Read the model definition and answer for the solid it produces. Units are mm, in the model's axes. Face numbers are marked on the shaded views. A direction names the side the tool comes from. Give positions to 0.01 mm unless a question says otherwise; leave off trailing zeros. Order: outer loops, then holes, each group sorted by start corner. A loop starts at its lowest first (then second) coordinate and runs counter-clockwise, first axis right, second up.
```python
from build123d import *

# Parameters (mm, degrees)
SCHIZZO2_W                                           = 51.888116
SCHIZZO2_H                                           = 40
ESTRUSIONE_ESTRUSIONE2_DEPTH                         = 10
ESTRUSIONE_ESTRUSIONE3_DEPTH                         = 12.5
ESTRUSIONE_ESTRUSIONE3_DEPTH_BACK                    = 10
SCHIZZO3_R                                           = 113
SCHIZZO3_R_2                                         = 105
SCHIZZO3_R_3                                         = 95
SCHIZZO3_R_4                                         = 92.5
TAGLIO_ESTRUSIONE1_DEPTH                             = 4.5
TAGLIO_ESTRUSIONE1_DEPTH_BACK                        = 4.5
SCHIZZO3_3_R                                         = 115
SCHIZZO3_3_R_2                                       = 113
SCHIZZO3_3_R_3                                       = 105
SCHIZZO3_3_R_4                                       = 95
TAGLIO_ESTRUSIONE2_DEPTH                             = 12.5
TAGLIO_ESTRUSIONE2_DEPTH_BACK                        = 12.5
SCHIZZO3_4_R                                         = 121.5
SCHIZZO3_4_R_2                                       = 115
TAGLIO_ESTRUSIONE3_DEPTH                             = 79.5
TAGLIO_ESTRUSIONE3_DEPTH_BACK                        = 79.5
ESTRUSIONE_ESTRUSIONE5_DEPTH                         = 51.888111
FORO_LAMATO_PER_VITE_M4_A_TESTA_CILINDRI_D           = 4.5
FORO_LAMATO_PER_VITE_M4_A_TESTA_CILINDRI_DEPTH       = 30
FORO_LAMATO_PER_VITE_M4_A_TESTA_CILINDRI_CBORE_D     = 10
FORO_LAMATO_PER_VITE_M4_A_TESTA_CILINDRI_CBORE_DEPTH = 2.6
FORO_LAMATO_PER_VITE_M4_A_TESTA_CILINDRI_TIP         = 1.351936393
SCHIZZO10_W                                          = 2
SCHIZZO10_H                                          = 17
TAGLIO_ESTRUSIONE4_DEPTH                             = 10
TAGLIO_ESTRUSIONE5_DEPTH                             = 33
RACCORDO1_R                                          = 10


with BuildPart() as part:
    # Schizzo2 → Estrusione-Estrusione2 (new body)
    with BuildSketch(Plane(origin=(0, 0, 0), x_dir=(1, 0, 0), z_dir=(0, 1, 0))):
        with Locations((-97.308977, 0)):
            Rectangle(SCHIZZO2_W, SCHIZZO2_H)
    extrude(amount=-ESTRUSIONE_ESTRUSIONE2_DEPTH)

    # Schizzo3 → Estrusione-Estrusione3 (add, two sides: drawn at the far end of the back side and taken through both)
    # profile 1 of 3: a face of its own
    with BuildSketch(Plane.XY.offset(-ESTRUSIONE_ESTRUSIONE3_DEPTH_BACK)):
        with Locations((0, 44)):
            Circle(SCHIZZO3_R)
        with Locations((0, 44)):
            Circle(SCHIZZO3_R_2, mode=Mode.SUBTRACT)
    # profile 2 of 3: a face of its own
    with BuildSketch(Plane.XY.offset(-ESTRUSIONE_ESTRUSIONE3_DEPTH_BACK)):
        with Locations((0, 44)):
            Circle(SCHIZZO3_R_2)
        with Locations((0, 44)):
            Circle(SCHIZZO3_R_3, mode=Mode.SUBTRACT)
    # profile 3 of 3: a face of its own
    with BuildSketch(Plane.XY.offset(-ESTRUSIONE_ESTRUSIONE3_DEPTH_BACK)):
        with Locations((0, 44)):
            Circle(SCHIZZO3_R_3)
        with Locations((0, 44)):
            Circle(SCHIZZO3_R_4, mode=Mode.SUBTRACT)
    extrude(amount=ESTRUSIONE_ESTRUSIONE3_DEPTH + ESTRUSIONE_ESTRUSIONE3_DEPTH_BACK)

    # Schizzo3<3> → Taglio-Estrusione1 (cut, two sides: drawn at the far end of the back side and taken through both)
    # profile 1 of 3: a face of its own
    with BuildSketch(Plane.XY.offset(-TAGLIO_ESTRUSIONE1_DEPTH_BACK)):
        with Locations((0, 44)):
            Circle(SCHIZZO3_3_R)
        with Locations((0, 44)):
            Circle(SCHIZZO3_3_R_2, mode=Mode.SUBTRACT)
    # profile 2 of 3: a face of its own
    with BuildSketch(Plane.XY.offset(-TAGLIO_ESTRUSIONE1_DEPTH_BACK)):
        with Locations((0, 44)):
            Circle(SCHIZZO3_3_R_2)
        with Locations((0, 44)):
            Circle(SCHIZZO3_3_R_3, mode=Mode.SUBTRACT)
    # profile 3 of 3: a face of its own
    with BuildSketch(Plane.XY.offset(-TAGLIO_ESTRUSIONE1_DEPTH_BACK)):
        with Locations((0, 44)):
            Circle(SCHIZZO3_3_R_3)
        with Locations((0, 44)):
            Circle(SCHIZZO3_3_R_4, mode=Mode.SUBTRACT)
    extrude(amount=TAGLIO_ESTRUSIONE1_DEPTH + TAGLIO_ESTRUSIONE1_DEPTH_BACK, mode=Mode.SUBTRACT)

    # Schizzo3<4> → Taglio-Estrusione2 (cut, two sides: drawn at the far end of the back side and taken through both)
    with BuildSketch(Plane.XY.offset(-TAGLIO_ESTRUSIONE2_DEPTH_BACK)):
        with Locations((0, 44)):
            Circle(SCHIZZO3_4_R)
        with Locations((0, 44)):
            Circle(SCHIZZO3_4_R_2, mode=Mode.SUBTRACT)
    extrude(amount=TAGLIO_ESTRUSIONE2_DEPTH + TAGLIO_ESTRUSIONE2_DEPTH_BACK, mode=Mode.SUBTRACT)

    # Schizzo4 → Taglio-Estrusione3 (cut, two sides: drawn at the far end of the back side and taken through both)
    with BuildSketch(Plane.XY.offset(12.5).offset(-TAGLIO_ESTRUSIONE3_DEPTH_BACK)):
        Polygon((150, 13), (150, -10), (150, -80), (-150, -80), (-150, -10), (0, -10), (0, 13), (-150, 13), (-150, 163), (150, 163), align=None)
    extrude(amount=TAGLIO_ESTRUSIONE3_DEPTH + TAGLIO_ESTRUSIONE3_DEPTH_BACK, mode=Mode.SUBTRACT)

    # Smusso1
    # the kernel refuses this chamfer: 4.942054941, 3 mm, written as the material it takes off along each edge
    with BuildSketch(Plane(origin=(-87.150731494, 13, 24.790313744), x_dir=(-0.998955732576957, 0.045688558213574655, 0), z_dir=(0, 0, -1))) as smusso1_piece_1:
        with BuildLine():
            Line((3.009603279, 0), (-2.049272113, -4.468643386))
            Line((-2.049272113, -4.468643386), (-2.138755111, -4.426662964))
            ThreePointArc((-2.138755111, -4.426662964), (-1.049342002, -2.223465239), (-0.091514438, 0.037345286))
            Line((-0.091514438, 0.037345286), (0.004515907, 0.098737882))
            ThreePointArc((0.004515907, 0.098737882), (1.506176357, 0.030057461), (3.014119187, 0.098737882))
            Line((3.014119187, 0.098737882), (3.009603279, 0))
        make_face()
    extrude(amount=47.080627488, mode=Mode.SUBTRACT)
    # the kernel refuses this chamfer: 4.942054941, 3 mm, written as the material it takes off along each edge
    with BuildSketch(Plane(origin=(-116.379670622, 13, -10), x_dir=(0, -0.9996219169112969, -0.02749587661058621), z_dir=(1, 0, 0))) as smusso1_2_piece_1:
        with BuildLine():
            Line((3.086019586, 0), (-0.169641465, -3.081353381))
            Line((-0.169641465, -3.081353381), (-0.22961878, -3.079703628))
            ThreePointArc((-0.22961878, -3.079703628), (-0.102387681, -1.540193489), (-0.059977315, 0.001649753))
            Line((-0.059977315, 0.001649753), (0.001649753, 0.059977315))
            ThreePointArc((0.001649753, 0.059977315), (1.543492994, 0.017566949), (3.087669338, 0.059977315))
            Line((3.087669338, 0.059977315), (3.086019586, 0))
        make_face()
    extrude(amount=34.07955152, mode=Mode.SUBTRACT)
    with BuildSketch(Plane(origin=(-116.379670622, 13, 12.5), x_dir=(0, -0.9996219169112969, 0.02749587661058621), z_dir=(1, 0, 0))) as smusso1_2_piece_2:
        with BuildLine():
            Line((3.086019586, 0), (-0.169641465, 3.081353381))
            Line((-0.169641465, 3.081353381), (-0.22961878, 3.079703628))
            ThreePointArc((-0.22961878, 3.079703628), (-0.102387681, 1.540193489), (-0.059977315, -0.001649753))
            Line((-0.059977315, -0.001649753), (0.001649753, -0.059977315))
            ThreePointArc((0.001649753, -0.059977315), (1.543492994, -0.017566949), (3.087669338, -0.059977315))
            Line((3.087669338, -0.059977315), (3.086019586, 0))
        make_face()
    extrude(amount=34.07955152, mode=Mode.SUBTRACT)

    # Schizzo7 → Estrusione-Estrusione5 (add)
    with BuildSketch(Plane(origin=(-71.364919, 0, 0), x_dir=(0, 0, -1), z_dir=(1, 0, 0))):
        Polygon((-20, 0), (-35, 0), (-35, 4), (-20, 4), (-14, 0), align=None)
        Polygon((20, 4), (35, 4), (35, 0), (20, 0), (14, 0), align=None)
    extrude(amount=-ESTRUSIONE_ESTRUSIONE5_DEPTH)

    # Foro lamato per Vite M4 a testa cilindrica piana-1
    with Locations(Plane(origin=(0, 4, 0), x_dir=(1, 0, 0), z_dir=(0, 1, 0))):
        with Locations((-97.308977, -27.5), (-97.308977, 27.5)):
            CounterBoreHole(FORO_LAMATO_PER_VITE_M4_A_TESTA_CILINDRI_D / 2, FORO_LAMATO_PER_VITE_M4_A_TESTA_CILINDRI_CBORE_D / 2, FORO_LAMATO_PER_VITE_M4_A_TESTA_CILINDRI_CBORE_DEPTH, depth=FORO_LAMATO_PER_VITE_M4_A_TESTA_CILINDRI_DEPTH)
            with Locations((0, 0, -(FORO_LAMATO_PER_VITE_M4_A_TESTA_CILINDRI_DEPTH + FORO_LAMATO_PER_VITE_M4_A_TESTA_CILINDRI_TIP / 2))):  # 118° drill point
                Cone(0, FORO_LAMATO_PER_VITE_M4_A_TESTA_CILINDRI_D / 2, FORO_LAMATO_PER_VITE_M4_A_TESTA_CILINDRI_TIP, mode=Mode.SUBTRACT)

    # Schizzo10 → Taglio-Estrusione4 (cut)
    with BuildSketch(Plane(origin=(0, 0, 0), x_dir=(1, 0, 0), z_dir=(0, 1, 0))):
        with Locations((-116.253035279, 0)):
            Rectangle(SCHIZZO10_W, SCHIZZO10_H)
    extrude(amount=-TAGLIO_ESTRUSIONE4_DEPTH, mode=Mode.SUBTRACT)

    # Schizzo11 → Taglio-Estrusione5 (cut)
    with BuildSketch(Plane(origin=(0, 4, 0), x_dir=(1, 0, 0), z_dir=(0, 1, 0))):
        Polygon((-123.253035, 14), (-123.253035, 35), (-104.808977, 35), (-114.808977, 14), align=None)
        Polygon((-89.808977, 35), (-71.364919, 35), (-71.364919, 14), (-79.808977, 14), align=None)
        Polygon((-123.253035, -14), (-123.253035, -35), (-104.808977, -35), (-114.808977, -14), align=None)
        Polygon((-89.808977, -35), (-71.364919, -35), (-71.364919, -14), (-79.808977, -14), align=None)
    extrude(amount=-TAGLIO_ESTRUSIONE5_DEPTH, mode=Mode.SUBTRACT)

    # Raccordo1
    raccordo1_edges = [part.edges().sort_by_distance(p)[0] for p in [
        (-104.808977, 2, -35),
        (-89.808977, 2, -35),
        (-104.808977, 2, 35),
        (-89.808977, 2, 35),
    ]]
    fillet(raccordo1_edges, radius=RACCORDO1_R)


solid = part.part
```
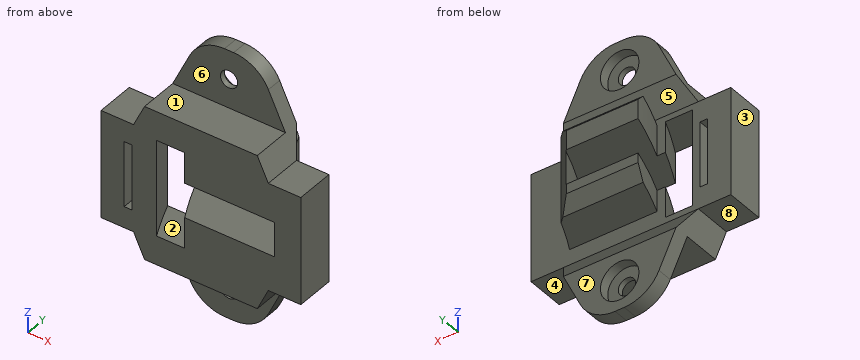
1) A tool of negligible diameter and unlimited length cuts with its end or side. For the marked faces 4, 5, 6, 7 and 8, from which of +Z, -Z, +X, -X, +Y, -Y can it reach the whole face along a straight path? Write none if from no direction.
Final values:
face 4: -Z, +X, +Y, -Y
face 5: +X, -X, +Y
face 6: +Z, +X, -X, -Y
face 7: -Z, +X, -X, +Y
face 8: -Z, -X, +Y, -Y
2) The part is cut by section C-C on z = -28.5. Determine the outline of the cut face in (x, y).
Final values:
outline: (-107.9, 0) - (-99.32, 0) - (-99.32, 1.4) - (-102.21, 1.4) - (-102.21, 4) - (-107.9, 4) - close; (-95.29, 0) - (-86.71, 0) - (-86.71, 4) - (-92.41, 4) - (-92.41, 1.4) - (-95.29, 1.4) - close
3) The part is cut by section D-D on y = -2. Determine the outline of the cut face in (x, z).
Final values:
outline: (-123.25, -14) - (-114.81, -14) - (-111.95, -20) - (-82.67, -20) - (-79.81, -14) - (-71.36, -14) - (-71.36, 14) - (-79.81, 14) - (-82.67, 20) - (-111.95, 20) - (-114.81, 14) - (-123.25, 14) - close; hole (-117.25, -8.5) - (-115.25, -8.5) - (-115.25, 8.5) - (-117.25, 8.5) - close; hole (-112.46, -12.5) - (-105.4, -12.5) - (-105.4, -4.5) - (-83.12, -4.5) - (-83.12, 4.5) - (-105.4, 4.5) - (-105.4, 12.5) - (-112.46, 12.5) - close
4) For a pull along X with two mould halves and no side action, classify the marked faces 1, 2 and 3 as released by +X, released by -X, zero draft, split by the parting line, or undercut.
Final values:
face 1: zero draft
face 2: undercut
face 3: released by -X
5) Consider L1, parallel to Z at x = -105.5, y = 7; L2, parallel to Z at x = -98.5, y = -5; L3, parallel to Z at x = -83, y = 2.25 (3 decimals). Determine where each line is inside the solid, lowest interval first.
Final values:
L1: z = -10 to -4.5, 4.5 to 12.5
L2: z = -20 to -4.5, 4.5 to 20
L3: z = -20.701 to -17.375, -10 to 12.5, 17.375 to 20.701
6) The part is cut by section A-A on y = 3. Determine the outline of the cut face in (x, z), and give its area (3 significant figures).
Final values:
outline: (-112.67, -18.5) - (-107.52, -29.3) arc R10 ccw to (-98.49, -35) - (-96.12, -35) arc R10 ccw to (-87.09, -29.3) - (-81.95, -18.5) - close; (-112.67, 18.5) - (-81.95, 18.5) - (-87.09, 29.3) arc R10 ccw to (-96.12, 35) - (-98.49, 35) arc R10 ccw to (-107.52, 29.3) - close; (-105.3, -10) - (-82.92, -10) - (-82.92, 12.5) - (-105.3, 12.5) - (-105.3, 4.5) - (-85.7, 4.5) - (-85.7, -4.5) - (-105.3, -4.5) - close; hole circle Ø10 at (-97.31, -27.5); hole circle Ø10 at (-97.31, 27.5)
area: 897 mm2
7) Given pin 1 (16.5 mm diameter, centred on x = -98, z = -24, fed in from +Y); pin 2 (1.5 mm diameter, centred on x = -83.5, z = -3.5, fed in from -Y); pin 3 (9.5 mm diameter, centred on x = -120, y = -7, fed in from +Z), each flat-ended and moving along its own axis, determine where each tip first touches the part or whether it passes through.
Final values:
pin 1: stops at y = 4
pin 2: stops at y = -2.66
pin 3: stops at z = 14
